Geometry: see drawing. Coordinates: mm, zero at the bounding-box minimum. Coordinates: 2 decimals unless noted, no trailing zeros. Write each loop counter-clockwise with the first axis right and the second up, starting at its lowest first coordinate (ties: lowest second). Pieces come first, ordered by that corner, then holes. Notation, with made-up numbers: (49, 17) -> (96, 17) arc R30 cw to (96, 45) -> close; hole circle Ø6 at (68, 25). An arc over 180 degrees is marked (long way). Answer as a JSON object with one key per item and string values. Group by question number.
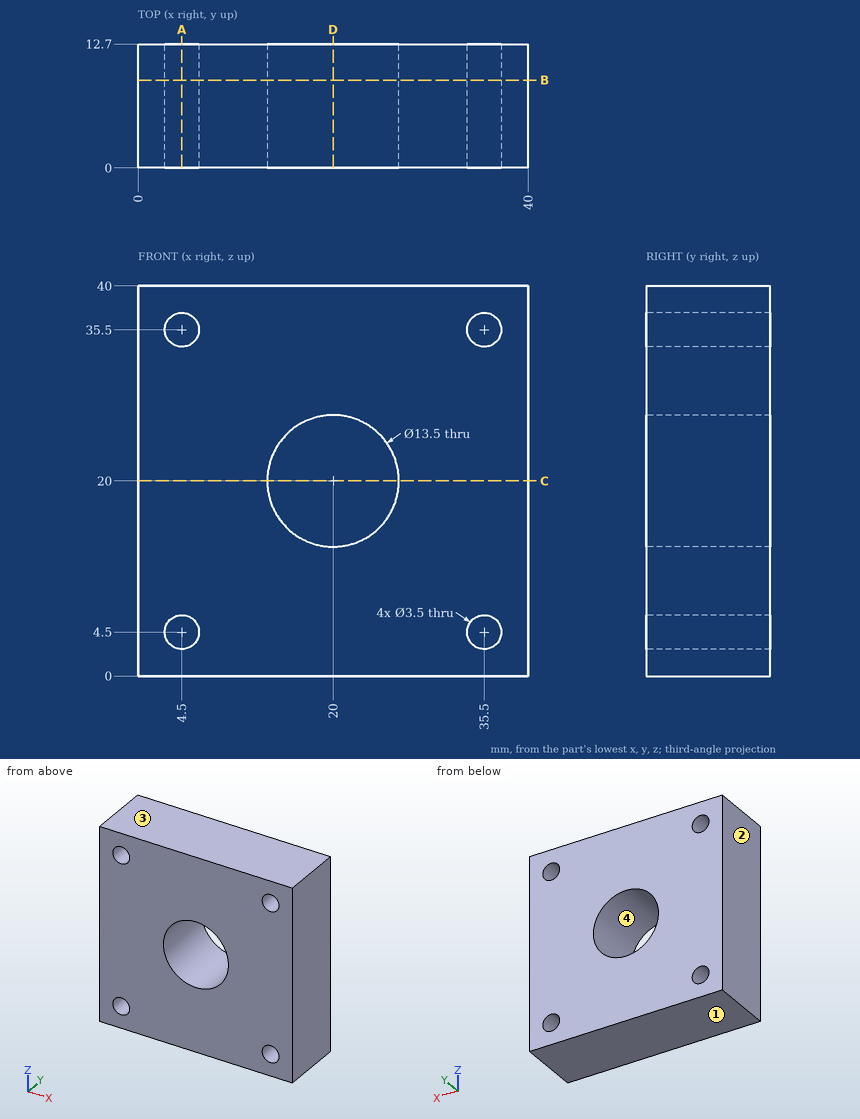
Item 1: Section A-A on x = 4.5. Output: boundary loops of the cut face in (y, z).
Item 2: Section D-D on x = 20. Output: boundary loops of the cut face in (y, z).
Item 3: Ray query, L1, parallel to Z at x = 4.5, y = 4.75; L2, parallel to X at y = 10.5, z = 35; L3, parallel to Z at x = 34, y = 10.5. Return the intervals inside material, ascending. Write a range as [from, to].
Item 4: Section C-C on z = 20. Output: boundary loops of the cut face in (x, y).
Item 5: Mould query, pull axis Z, two halves, no side actions, for the marked faces 1, 2, 3 and 4. Classes: +Z half, -Z half, draft (parallel to the pull), parting line (faces both ways), or undercut.
Item 6: Section B-B on y = 9. Output: boundary loops of the cut face in (x, z), then the cut area to 3 significant figures.
Answer sheet:
{
 "1": {"outline": "(0, 0) -> (12.7, 0) -> (12.7, 2.75) -> (0, 2.75) -> close; (0, 6.25) -> (12.7, 6.25) -> (12.7, 33.75) -> (0, 33.75) -> close; (0, 37.25) -> (12.7, 37.25) -> (12.7, 40) -> (0, 40) -> close"},
 "2": {"outline": "(0, 0) -> (12.7, 0) -> (12.7, 13.25) -> (0, 13.25) -> close; (0, 26.75) -> (12.7, 26.75) -> (12.7, 40) -> (0, 40) -> close"},
 "3": {"L1": "z = [0, 2.75], [6.25, 33.75], [37.25, 40]", "L2": "x = [0, 2.82], [6.18, 33.82], [37.18, 40]", "L3": "z = [0, 3.6], [5.4, 34.6], [36.4, 40]"},
 "4": {"outline": "(0, 0) -> (13.25, 0) -> (13.25, 12.7) -> (0, 12.7) -> close; (26.75, 0) -> (40, 0) -> (40, 12.7) -> (26.75, 12.7) -> close"},
 "5": {"face 1": "-Z half", "face 2": "draft", "face 3": "+Z half", "face 4": "undercut"},
 "6": {"outline": "(0, 0) -> (40, 0) -> (40, 40) -> (0, 40) -> close; hole circle Ø3.5 at (4.5, 4.5); hole circle Ø3.5 at (4.5, 35.5); hole circle Ø13.5 at (20, 20); hole circle Ø3.5 at (35.5, 4.5); hole circle Ø3.5 at (35.5, 35.5)", "area": "1,420 mm^2"}
}
